from build123d import *

# Parameters (mm, degrees)
F1_W           = 76.2
F1_H           = 63.5
F2_DEPTH       = 6.35
F4_D           = 11.303
F4_CBORE_D     = 21.717
F4_CBORE_DEPTH = 3.302
F6_D           = 6.985
F7_D           = 6.985
F8_D           = 5.207
F9_D           = 5.207
F10_D          = 5.207
F11_R          = 6.35


with BuildPart() as f2:
    # F1 (on Top) → F2 (new body)
    with BuildSketch(Plane.XY):
        Rectangle(F1_W, F1_H)
    extrude(amount=F2_DEPTH)

    # F4 (through all)
    with Locations(Plane.XY.offset(6.35)):
        with Locations((0, 0)):
            CounterBoreHole(F4_D / 2, F4_CBORE_D / 2, F4_CBORE_DEPTH)

    # F6 (through all)
    with Locations(Plane.XY.offset(6.35)):
        with Locations((-28.067, 0)):
            Hole(F6_D / 2)

    # F7 (through all)
    with Locations(Plane.XY.offset(6.35)):
        with Locations((28.067, 0)):
            Hole(F7_D / 2)

    # F8 (through all)
    with Locations(Plane(origin=(0, 0, 0), x_dir=(1, 0, 0), z_dir=(0, 0, -1))):
        with Locations((-23.622, 23.622)):
            Hole(F8_D / 2)

    # F9 (through all)
    with Locations(Plane(origin=(0, 0, 0), x_dir=(1, 0, 0), z_dir=(0, 0, -1))):
        with Locations((23.622, 23.622), (-23.622, -23.622)):
            Hole(F9_D / 2)

    # F10 (through all)
    with Locations(Plane(origin=(0, 0, 0), x_dir=(1, 0, 0), z_dir=(0, 0, -1))):
        with Locations((23.622, -23.622)):
            Hole(F10_D / 2)

    # F11
    f11_edges = [f2.edges().sort_by_distance(p)[0] for p in [
        (-38.1, -31.75, 3.175),
        (38.1, -31.75, 3.175),
        (38.1, 31.75, 3.175),
        (-38.1, 31.75, 3.175),
    ]]
    fillet(f11_edges, radius=F11_R)


solid = f2.part
The listing builds one solid part. Answer for the finished solid, in the listing's coordinates (mm). A direction names the side the tool comes from. Give positions to 0.01 mm unless a question says otherwise; leave off trailing zeros. Write each loop counter-clockwise with the first axis right and the second up, starting at its lowest first coordinate (ties: lowest second). Pieces come first, ordered by that corner, then holes. Notation, with made-up numbers: (-29, 74.5) -> (21, 74.5) arc R15 ccw to (21, 93.5) -> close; hole circle Ø1 at (12.25, 15.25). An arc over 180 degrees is marked (long way). Use a Markdown table: item, result.
(1) Find the intervals of material crossed by probe 1 along Y at (x, z) = (0, 5.2); probe 2 along X at (y, z) = (-0.5, 2.5); probe 3 along X at (y, z) = (-1.5, 4.25), in increasing order. Write a range as from..to.
Return value:
| item | result |
|---|---|
| probe 1 | -31.75..-10.86, 10.86..31.75 |
| probe 2 | -38.1..-31.52, -24.61..-5.63, 5.63..24.61, 31.52..38.1 |
| probe 3 | -38.1..-31.22, -24.91..-10.75, 10.75..24.91, 31.22..38.1 |
(2) Section B-B, the plane x = 0 is taken. Determine the outline of the cut face in (y, z).
Return value:
| item | result |
|---|---|
| outline | (-31.75, 0) -> (-5.65, 0) -> (-5.65, 3.05) -> (-10.86, 3.05) -> (-10.86, 6.35) -> (-31.75, 6.35) -> close; (5.65, 0) -> (31.75, 0) -> (31.75, 6.35) -> (10.86, 6.35) -> (10.86, 3.05) -> (5.65, 3.05) -> close |
(3) Determine the mould class of faces 3 (the flat face through (-38.1, 0, 3)), 4 (the flat face through (-1, -7, 0)), 5 (the cylindrical face through (-21.56, 25.21, 3.22)) for opening direction X: released by +X, released by -X, zero draft, split by the parting line, or undercut.
Return value:
| item | result |
|---|---|
| face 3 | released by -X |
| face 4 | zero draft |
| face 5 | undercut |
(4) Section C-C, the plane z = 2 is taken. Give the number of separate pieces and of enclosed holes in the cut face, then the cut area to 3 significant figures.
Return value:
| item | result |
|---|---|
| separate pieces | 1 |
| enclosed holes | 7 |
| area | 4,540 mm2 |
(5) For faces 1 (the cylindrical face through (-2.35, -10.6, 4.72)), 2 (the flat face through (38.1, 0, 3)), determine the directions among +Z, -Z, +X, -X, +Y, -Y from which every point of the face is accessible in a straight line to the end or side of a thin tool.
Return value:
| item | result |
|---|---|
| face 1 | +Z |
| face 2 | +Z, -Z, +X, +Y, -Y |
(6) Section A-A, the plane y = 0 is taken. Determine the outline of the cut face in (x, z), then the cut area to 3 significant figures.
Return value:
| item | result |
|---|---|
| outline | (-38.1, 0) -> (-31.56, 0) -> (-31.56, 6.35) -> (-38.1, 6.35) -> close; (-24.57, 0) -> (-5.65, 0) -> (-5.65, 3.05) -> (-10.86, 3.05) -> (-10.86, 6.35) -> (-24.57, 6.35) -> close; (5.65, 0) -> (24.57, 0) -> (24.57, 6.35) -> (10.86, 6.35) -> (10.86, 3.05) -> (5.65, 3.05) -> close; (31.56, 0) -> (38.1, 0) -> (38.1, 6.35) -> (31.56, 6.35) -> close |
| area | 289 mm2 |
(7) Flat-ended cylindrical pins translate along their axes: P1, Ø3, axis at x = -23.622, y = -23.622, coming from the -Z side; P2, Ø11, axis at x = 1, y = -3.5, coming from the +Z side. Find the tip coordinate at first contact, or state that the pin passes through.
Return value:
| item | result |
|---|---|
| P1 | through |
| P2 | z = 3.05 |
